The figure shows three views and two pictorial views of one solid part (mm, origin at its lowest corner). Answer the questions. A direction names the side the tool comes from. Give positions to 0.01 mm unless a question says otherwise; leave off trailing zeros. Order: outer loops, then holes, each group sorted by start corner. A loop starts at its lowest first (then second) coordinate and runs counter-clockwise, first axis right, second up. Notation, with made-up numbers: (-24, -10) - (-5, -10) arc R20 ccw to (-5, 13) - close; hole circle Ø3 at (51.5, 87). An arc over 180 degrees is marked (long way). Write item = value, one per line.
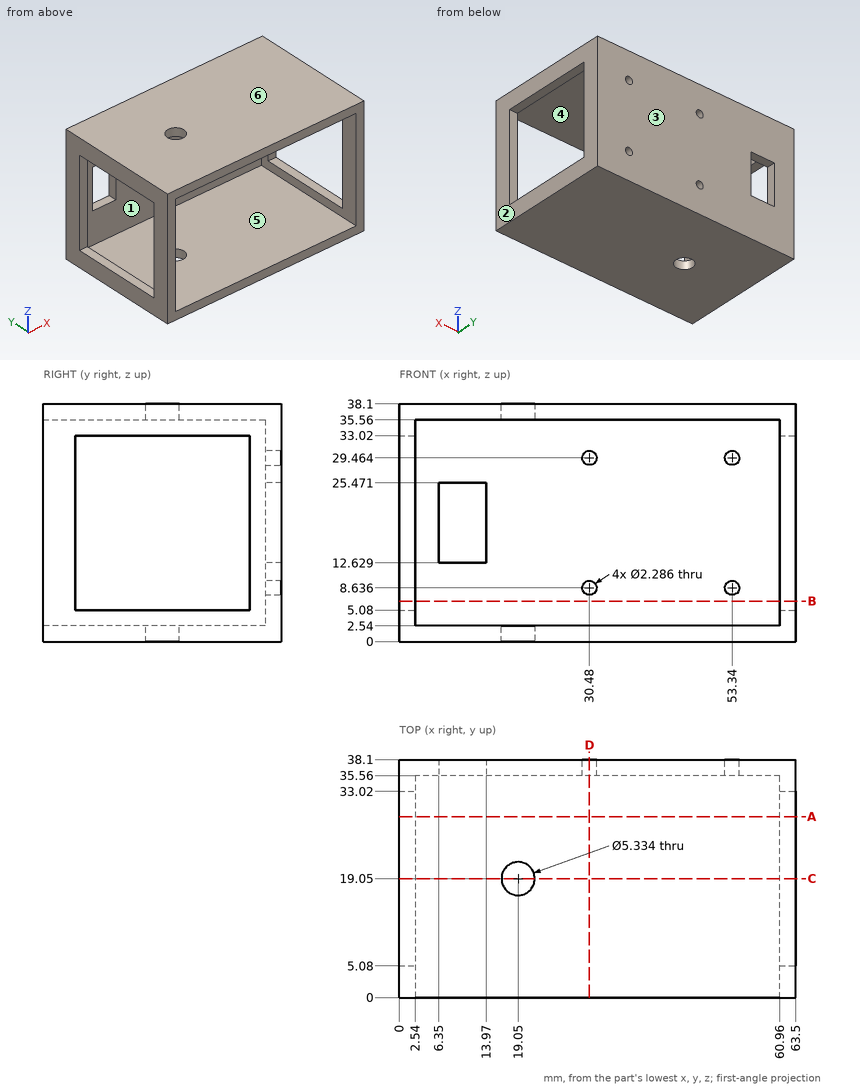
1. Determine the mould class of the marked faces 3, 4, 5 and 6 for opening direction Z: +Z half, -Z half, draft (parallel to the pull), parting line (faces both ways), or undercut.
Recorded:
face_3 = draft
face_4 = undercut
face_5 = undercut
face_6 = +Z half
2. Straight lines are drawn through the part: L1, parallel to Z at x = 53.34, y = 36.75; L2, parallel to X at y = 26, z = 3.5; L3, parallel to Z at x = 7.5, y = 12. For each, find the intervals that lie inside material, in ascending order. Write a range as [from, to].
Recorded:
L1 = [0, 7.49], [9.78, 28.32], [30.61, 38.1]
L2 = [0, 2.54], [60.96, 63.5]
L3 = [0, 2.54], [35.56, 38.1]
3. A flat-ended cylindrical pin translates along its axis: pin 1 (1 mm diameter, centred on x = 52.5, z = 22, fed in from -Y). Find the tip coordinate at first contact, or state that the pin passes through.
Recorded:
pin_1 = 35.56
4. Section D-D (x = 30.48) is taken. Determine the outline of the cut face in (y, z).
Recorded:
outline = (0, 0) - (38.1, 0) - (38.1, 7.49) - (35.56, 7.49) - (35.56, 2.54) - (0, 2.54) - close; (0, 35.56) - (35.56, 35.56) - (35.56, 30.61) - (38.1, 30.61) - (38.1, 38.1) - (0, 38.1) - close; (35.56, 9.78) - (38.1, 9.78) - (38.1, 28.32) - (35.56, 28.32) - close
5. Section B-B (z = 6.5) is taken. Determine the outline of the cut face in (x, y), and give its area (3 significant figures).
Recorded:
outline = (0, 0) - (2.54, 0) - (2.54, 5.08) - (0, 5.08) - close; (0, 33.02) - (2.54, 33.02) - (2.54, 35.56) - (60.96, 35.56) - (60.96, 33.02) - (63.5, 33.02) - (63.5, 38.1) - (0, 38.1) - close; (60.96, 0) - (63.5, 0) - (63.5, 5.08) - (60.96, 5.08) - close
area = 200 mm^2
6. For the marked faces 1 and 2, determine the directions among +Z, -Z, +X, -X, +Y, -Y from which every point of the face is accessible in a straight line to the end or side of a thin tool.
Recorded:
face_1 = -Y
face_2 = +Z, -Z, +X, +Y, -Y
7. Section A-A (y = 29) is taken. Determine the outline of the cut face in (x, z), and give its area (3 significant figures).
Recorded:
outline = (0, 0) - (63.5, 0) - (63.5, 5.08) - (60.96, 5.08) - (60.96, 2.54) - (2.54, 2.54) - (2.54, 5.08) - (0, 5.08) - close; (0, 33.02) - (2.54, 33.02) - (2.54, 35.56) - (60.96, 35.56) - (60.96, 33.02) - (63.5, 33.02) - (63.5, 38.1) - (0, 38.1) - close
area = 348 mm^2
8. Section C-C (y = 19.05) is taken. Determine the outline of the cut face in (x, z), and give its area (3 significant figures).
Recorded:
outline = (0, 0) - (16.38, 0) - (16.38, 2.54) - (2.54, 2.54) - (2.54, 5.08) - (0, 5.08) - close; (0, 33.02) - (2.54, 33.02) - (2.54, 35.56) - (16.38, 35.56) - (16.38, 38.1) - (0, 38.1) - close; (21.72, 0) - (63.5, 0) - (63.5, 5.08) - (60.96, 5.08) - (60.96, 2.54) - (21.72, 2.54) - close; (21.72, 35.56) - (60.96, 35.56) - (60.96, 33.02) - (63.5, 33.02) - (63.5, 38.1) - (21.72, 38.1) - close
area = 321 mm^2
